Autodesk Inventor part; units mm, degrees
ref_plane "YZ Plane" through (0, 0, 0) normal (1, 0, 0) x (0, 1, 0)
ref_plane "XZ Plane" through (0, 0, 0) normal (0, 1, 0) x (-1, 0, 0)
ref_plane "XY Plane" through (0, 0, 0) normal (0, 0, 1) x (1, 0, 0)
sketch "Sketch1" plane through (0, 0, 0) normal (0, 0, 1) x (1, 0, 0)
  circle A0 centre (0, 0) radius 11.1125
  circle A1 centre (22.86, 0) radius 9.525
  arc A2 (-3.7868, 13.7765) -> (-3.7868, -13.7765) centre (0, 0) ccw
  circle A3 centre (22.86, -25.4) radius 2.5797
  circle A4 centre (22.86, 0) radius 25.4 construction
  circle A5 centre (48.26, 0) radius 2.5797
  circle A6 centre (22.86, 25.4) radius 2.5797
  circle A7 centre (22.86, 0) radius 29.9974
  dimension "d0" = 22.225
  dimension "d1" = 19.05
  dimension "d2" = 22.86
  dimension "d3" = 3.175
  dimension "d8" = 50.8
  dimension "d11" = 5.1594
  dimension "d17" = 59.9948
extrude "Extrusion1" add sketch "Sketch1" along normal blind 6.985 contours A0 A7 | A0 A7 A2 picked at (30.9689, 18.7513)
sketch "Sketch2" plane through (0, 0, 6.985) normal (0, 0, 1) x (1, 0, 0)
  circle A0 centre (0, 0) radius 11.1125
  circle A1 centre (0, 0) radius 8.5725
  dimension "d14" = 2.54
extrude "Extrusion2" add sketch "Sketch2" against normal blind 3.0226
fillet "Fillet1" radius 3.175 1 edges at (-14.2875, 0, 6.985)
properties part number "MotorBracket" material "ABS Plastic"
Design review of the part built by this model. Coordinates are the model's own, in mm. A direction names the side the tool comes from. Round coordinates to 2 decimals unless told otherwise and drop trailing zeros. Write each loop counter-clockwise with the first axis right and the second up, starting at its lowest first coordinate (ties: lowest second). Pieces come first, ordered by that corner, then holes. Notation, with made-up numbers: (42.25, 18) - (82.25, 18) arc R23 ccw to (82.25, 27) - close; hole circle Ø2 at (-28.75, 5). An arc over 180 degrees is marked (long way). Use a Markdown table: item, result. Add a question column.
1. We need section B-B (x = 22.86). State the section outline as (y, z) points (3 decimals).
2. We need section A-A (y = 0). Count the separate pieces of the cut face and the enclosed holes in it, then the cut area to 3 significant figures.
3. For faces 1 (the face through (6, -7, 3.962)), 2 (the face through (35, 0, 6.985)), list the 3-axis set-ups (+Z, -Z, +X, -X, +Y, -Y) from which the entire face can be reached by the end or side of a thin tool; tool diameter is ignored.
4. Clearance check with flat-ended pins moving along their axes: pin 1 (1.5 mm diameter, centred on y = -1.5, z = 1, fed in from -X); pin 2 (1 mm diameter, centred on x = 2.5, z = 5, fed in from -Y); pin 3 (18 mm diameter, centred on x = 1, y = 1, fed in from -Z). State where each tip first meets the part, or that it passes through.
5. Wall thickness on probe 1 along Y at (x, z) = (22.86, 3.75) (3 decimals); probe 2 along X at (y, z) = (-4.5, 2); probe 3 along X at (y, z) = (6.5, 5.75): over which ranges is each line inside the solid? List them lowest first.
6. We need section D-D (x = 30.5). State the section outline as (y, z) points (3 decimals).
7. Mouldability with a two-part tool opening along Y and no side actions: class faces 3 (the face through (52.834, 1.182, 3.444)), 4 (the face through (34, 0, 0)), 5 (the face through (50.721, -0.775, 3.444)) as +Y half, -Y half, draft (parallel to the pull), parting line (faces both ways), or undercut.
Output:
| question | item | result |
|---|---|---|
| 1 | outline | (-29.997, 0) - (-27.98, 0) - (-27.98, 6.985) - (-29.997, 6.985) - close; (-22.82, 0) - (-9.525, 0) - (-9.525, 6.985) - (-22.82, 6.985) - close; (9.525, 0) - (22.82, 0) - (22.82, 6.985) - (9.525, 6.985) - close; (27.98, 0) - (29.997, 0) - (29.997, 6.985) - (27.98, 6.985) - close |
| 2 | separate pieces | 4 |
| 2 | enclosed holes | 0 |
| 2 | area | 158 mm2 |
| 3 | face 1 | -Z |
| 3 | face 2 | +Z, +X, -X, +Y, -Y |
| 4 | pin 1 | stops at x = -14.27 |
| 4 | pin 2 | stops at y = -22.48 |
| 4 | pin 3 | stops at z = 3.96 |
| 5 | probe 1 | y = -29.997 to -27.98, -22.82 to -9.525, 9.525 to 22.82, 27.98 to 29.997 |
| 5 | probe 2 | x = -13.56 to -10.16, 10.16 to 14.47, 31.25 to 52.52 |
| 5 | probe 3 | x = -11.98 to -5.59, 5.59 to 15.9, 29.82 to 52.14 |
| 6 | outline | (-29.008, 0) - (-5.688, 0) - (-5.688, 6.985) - (-29.008, 6.985) - close; (5.688, 0) - (29.008, 0) - (29.008, 6.985) - (5.688, 6.985) - close |
| 7 | face 3 | parting line |
| 7 | face 4 | draft |
| 7 | face 5 | undercut |
